```python
from build123d import *

# Parameters (mm, degrees)
SKETCH_R        = 5
SKETCH_R_2      = 2.75
PAD_DEPTH       = 20
SKETCH001_R     = 3.3
POCKET_DEPTH    = 43.001
SKETCH002_R     = 5.4
POCKET001_DEPTH = 1.5
SKETCH003_R     = 13
POCKET002_DEPTH = 6
SKETCH004_R     = 13
POCKET003_DEPTH = 6


with BuildPart() as part:
    # Sketch → Pad (new body)
    with BuildSketch(Plane.XZ):
        Polygon((-30, 0), (30, 0), (30, 32.5), (17, 32.5), (17, 43), (-17, 43), (-17, 32.5), (-30, 32.5), align=None)
        with Locations((0, 25)):
            Circle(SKETCH_R, mode=Mode.SUBTRACT)
        with Locations((-23, 25)):
            Circle(SKETCH_R_2, mode=Mode.SUBTRACT)
        with Locations((-23, 7)):
            Circle(SKETCH_R_2, mode=Mode.SUBTRACT)
        with Locations((23, 7)):
            Circle(SKETCH_R_2, mode=Mode.SUBTRACT)
        with Locations((23, 25)):
            Circle(SKETCH_R_2, mode=Mode.SUBTRACT)
    extrude(amount=PAD_DEPTH)

    # Sketch001 (on Face1 of Pad) → Pocket (cut, through all)
    with BuildSketch(Plane(origin=(0, 0, 0), x_dir=(1, 0, 0), z_dir=(0, 0, -1))):
        with Locations((-23, 10)):
            Circle(SKETCH001_R)
        with Locations((23, 10)):
            Circle(SKETCH001_R)
    extrude(amount=-POCKET_DEPTH, mode=Mode.SUBTRACT)

    # Sketch002 (on Face9 of Pocket) → Pocket001 (cut)
    with BuildSketch(Plane(origin=(0, 0, 32.5), x_dir=(-1, 0, 0), z_dir=(0, 0, 1))):
        with Locations((-23, 10)):
            Circle(SKETCH002_R)
        with Locations((23, 10)):
            Circle(SKETCH002_R)
    extrude(amount=-POCKET001_DEPTH, mode=Mode.SUBTRACT)

    # Sketch003 (on Face4 of Pocket001) → Pocket002 (cut)
    with BuildSketch(Plane.XZ.offset(20)):
        with Locations((0, 25)):
            Circle(SKETCH003_R)
    extrude(amount=-POCKET002_DEPTH, mode=Mode.SUBTRACT)

    # Sketch004 (on Face3 of Pocket002) → Pocket003 (cut)
    with BuildSketch(Plane(origin=(0, 0, 0), x_dir=(1, 0, 0), z_dir=(0, 1, 0))):
        with Locations((0, -25)):
            Circle(SKETCH004_R)
    extrude(amount=-POCKET003_DEPTH, mode=Mode.SUBTRACT)


solid = part.part
```
Work out the finished part from the listing and answer in its coordinate system (mm). A direction names the side the tool comes from. Give positions to 0.01 mm unless a question says otherwise; leave off trailing zeros. Loops run counter-clockwise (first coordinate to the right, second up) from the corner with the lowest first, then second, coordinate; pieces in that order, holes last. Notation, with made-up numbers: (85.5, 81) - (118.5, 81) arc R11 cw to (118.5, 101) - close; hole circle Ø10 at (36, 28). An arc over 180 degrees is marked (long way). Use CSV: the item, a comma, the result in double quotes. Start each with the question number.
(1) Each of these flat-tipped pins is pushed along its axis until it touches: pin 1 (8.5 mm diameter, centred on x = -23, y = -10, fed in from +Z); pin 2 (10 mm diameter, centred on y = -17.5, z = 36, fed in from +X); pin 3 (3.5 mm diameter, centred on x = 23, z = 25, fed in from -Y); pin 4 (12 mm diameter, centred on x = 25.5, y = -11, fed in from +Z). Where does it stop, or does it pass through?
(2) A tool of negligible diameter and unlimited length cuts with its end or side. For faces 1 (the face through (17, -10, 38)), 2 (the face through (6.99, -17.04, 35.96)), 3 (the face through (6, -6, 25)), 4 (the face through (-23, -6, 31)), from which of +Z, -Z, +X, -X, +Y, -Y can it reach the whole face along a straight path? Write none if from no direction.
(3) Find section A-A, the plane z = 7. Determine the outline of the cut face in (x, y), plus the area to 3 significant figures.
(4) Find the intervals of material crossed by L1, parallel to Z at x = 23, y = -15; L2, parallel to X at y = -10, z = 17; L3, parallel to Z at x = 23, y = -2, in increasing order.
(5) Determine the mould class of faces 5 (the face through (23, -6, 31)), 6 (the face through (20.51, -5.21, 31.76)), 7 (the face through (6, -20, 12)), 8 (the face through (-20.38, -4.03, 25.83)) for opening direction Y: released by +Y, released by -Y, zero draft, split by the parting line, or undercut.
(6) Find section B-B, the plane x = 0. Determine the outline of the cut face in (y, z).
(7) Find section C-C, the plane x = -23. Determine the outline of the cut face in (y, z), plus the area to 3 significant figures.
(8) Find section D-D, the plane z = 25. Count the separate pieces of the cut face and the enclosed holes in it, plus the area to 3 significant figures.
Results found:
1,pin 1,"z = 31"
1,pin 2,"x = 30"
1,pin 3,"through"
1,pin 4,"z = 32.5"
2,face 1,"+Z, +X, +Y, -Y"
2,face 2,"-Y"
2,face 3,"+Y"
2,face 4,"+Z"
3,outline,"(-30, -20) - (-25.75, -20) - (-25.75, -11.82) arc R3.3 cw to (-25.75, -8.18) - (-25.75, 0) - (-30, 0) - close; (-20.25, -20) - (20.25, -20) - (20.25, -11.82) arc R3.3 cw to (20.25, -8.18) - (20.25, 0) - (-20.25, 0) - (-20.25, -8.18) arc R3.3 cw to (-20.25, -11.82) - close; (25.75, -20) - (30, -20) - (30, 0) - (25.75, 0) - (25.75, -8.18) arc R3.3 cw to (25.75, -11.82) - close"
3,area,"975 mm^2"
4,L1,"0 to 4.25, 9.75 to 22.25, 27.75 to 31"
4,L2,"-30 to -26.3, -19.7 to 19.7, 26.3 to 30"
4,L3,"0 to 4.25, 9.75 to 22.25, 27.75 to 32.5"
5,face 5,"undercut"
5,face 6,"undercut"
5,face 7,"released by -Y"
5,face 8,"zero draft"
6,outline,"(-20, 0) - (0, 0) - (0, 12) - (-6, 12) - (-6, 20) - (-14, 20) - (-14, 12) - (-20, 12) - close; (-20, 38) - (-14, 38) - (-14, 30) - (-6, 30) - (-6, 38) - (0, 38) - (0, 43) - (-20, 43) - close"
7,outline,"(-20, 0) - (-13.3, 0) - (-13.3, 4.25) - (-20, 4.25) - close; (-20, 9.75) - (-13.3, 9.75) - (-13.3, 22.25) - (-20, 22.25) - close; (-20, 27.75) - (-13.3, 27.75) - (-13.3, 31) - (-15.4, 31) - (-15.4, 32.5) - (-20, 32.5) - close; (-6.7, 0) - (0, 0) - (0, 4.25) - (-6.7, 4.25) - close; (-6.7, 9.75) - (0, 9.75) - (0, 22.25) - (-6.7, 22.25) - close; (-6.7, 27.75) - (0, 27.75) - (0, 32.5) - (-4.6, 32.5) - (-4.6, 31) - (-6.7, 31) - close"
7,area,"282 mm^2"
8,separate pieces,"4"
8,enclosed holes,"0"
8,area,"583 mm^2"
